from build123d import *

# Parameters (mm, degrees)
SKETCH2_W          = 20
SKETCH2_H          = 20
CUT_EXTRUDE1_DEPTH = 40


with BuildPart() as part:
    # Sketch1 → Revolve1 (revolve)
    with BuildSketch(Plane.XY, mode=Mode.PRIVATE) as revolve1_sk:
        Polygon((0, 0), (0, 5), (0.433012702, 5.75), (39.566987298, 5.75), (40, 5), (40, 0), align=None)
    revolve(revolve1_sk.sketch.rotate(Axis((40, 0, 0), (-1, 0, 0)), 270), axis=Axis((40, 0, 0), (-1, 0, 0)))

    # Sketch2 → Cut-Extrude1 (cut)
    with BuildSketch(Plane(origin=(0, 0, 0), x_dir=(0, 0, -1), z_dir=(1, 0, 0))):
        Rectangle(SKETCH2_W, SKETCH2_H)
        Polygon((-5, 2.886751346), (-5, -2.886751346), (0, -5.773502692), (5, -2.886751346), (5, 2.886751346), (0, 5.773502692), align=None, mode=Mode.SUBTRACT)
    extrude(amount=CUT_EXTRUDE1_DEPTH, mode=Mode.SUBTRACT)

    # Sketch3 → Cut-Revolve1 (revolve, cut)
    with BuildSketch(Plane.XY, mode=Mode.PRIVATE) as cut_revolve1_sk:
        Polygon((25.6, 0), (27.019415637, 2.4585), (39.4585, 2.4585), (40, 3), (40, 0), align=None)
    revolve(cut_revolve1_sk.sketch.rotate(Axis((40, 0, 0), (-1, 0, 0)), 270), axis=Axis((40, 0, 0), (-1, 0, 0)), mode=Mode.SUBTRACT)

    # Sketch4 → Revolve2 (revolve)
    with BuildSketch(Plane.XY, mode=Mode.PRIVATE) as revolve2_sk:
        Polygon((-9, 0), (-9, 2.4585), (-8.4585, 3), (-0.9, 3), (-0.9, 2.4585), (0, 2.4585), (0, 0), align=None)
    revolve(revolve2_sk.sketch.rotate(Axis((0, 0, 0), (-1, 0, 0)), 270), axis=Axis((0, 0, 0), (-1, 0, 0)))


solid = part.part
Geometry: final body of the model. Coordinates: model frame, mm. A direction names the side the tool comes from. Give positions to 0.01 mm unless a question says otherwise; leave off trailing zeros. Loops run counter-clockwise (first coordinate to the right, second up) from the corner with the lowest first, then second, coordinate; pieces in that order, holes last. Notation, with made-up numbers: (4, 43.5) - (41, 43.5) arc R20 ccw to (41, 77.5) - close; hole circle Ø9 at (-26, 75.25). An arc over 180 degrees is marked (long way). One line per question, with ' | ' between items. Start each with the question number.
(1) Section query A-A on x = 7. Return loops of the section in (y, z).
(2) Contact query for flat-ended pins moving along their axis: pin 1 (6 mm diameter, centred on x = 16.5, z = -3.5, fed in from -Y); pin 2 (4 mm diameter, centred on y = 0, z = 0, fed in from +X); pin 3 (1 mm diameter, centred on x = 7, z = 3, fed in from -Y). Output: stop coordinate, or through.
(3) Reachability of faces 1 (the flat face through (20, 0, 5)), 2 (the cylindrical face through (-4.63, 0.9, 2.86)) from +Z, -Z, +X, -X, +Y, -Y: full face, straight path, thin tool, end or side. Return the list, or none.
(4) Ray query, line 1 (Y direction, x = 30.75, z = 0); line 2 (X direction, y = -1.25, z = 3.75); line 3 (Z direction, x = -2, y = 0.25). Return the intervals inside material, ascending. Write a range as from..to.
(5) Pull-direction query (X, two-part tool) for faces 3 (the conical face through (0.12, 2.59, 4.52)), 4 (the conical face through (39.897, -2.6, 4.479)), 5 (the cylindrical face through (-0.444, 0.738, 2.345)), 6 (the cylindrical face through (33.326, 0.738, 2.345)); classes: released by +X, released by -X, zero draft, split by the parting line, or undercut.
(6) Section query B-B on x = -3. Return loops of the section in (y, z), then the cut area to 3 significant figures.
The answers:
1) outline: (-5.75, -0.04) - (-2.91, -4.96) arc R5.75 ccw to (-2.84, -5) - (2.84, -5) arc R5.75 ccw to (2.91, -4.96) - (5.75, -0.04) arc R5.75 ccw to (5.75, 0.04) - (2.91, 4.96) arc R5.75 ccw to (2.84, 5) - (-2.84, 5) arc R5.75 ccw to (-2.91, 4.96) - (-5.75, 0.04) arc R5.75 ccw to start
2) pin 1: y = -5.48 | pin 2: x = 26.75 | pin 3: y = -4.33
3) face 1: +Z, +X, -X, +Y, -Y | face 2: -X
4) line 1: -5.75..-2.46, 2.46..5.75 | line 2: 0..40 | line 3: -2.99..2.99
5) face 3: released by -X | face 4: released by +X | face 5: undercut | face 6: zero draft
6) outline: circle Ø6 at (0, 0) | area: 28.3 mm2
